from build123d import *

# Parameters (mm, degrees)
SKETCH2_R             = 6.35
SKETCH2_R_2           = 3.81
BOSS_EXTRUDE1_DEPTH   = 34.925
BOSS_EXTRUDE1_2_DEPTH = 34.925
BOSS_EXTRUDE1_3_DEPTH = 34.925
BOSS_EXTRUDE1_4_DEPTH = 34.925
SKETCH1_R             = 77.4954
SKETCH1_R_2           = 57.15
BOSS_EXTRUDE2_DEPTH   = 3.175
SKETCH3_R             = 3.81
CUT_EXTRUDE1_DEPTH    = 4.175
FILLET1_R             = 2.54


with BuildPart() as part:
    # Sketch2 → Boss-Extrude1 (new body)
    with BuildSketch(Plane(origin=(0, -40.33266, 0), x_dir=(1, 0, 0), z_dir=(0, 1, 0))):
        with Locations((-38.1, 56.870055469)):
            Circle(SKETCH2_R)
        with Locations((-38.1, 56.870055469)):
            Circle(SKETCH2_R_2, mode=Mode.SUBTRACT)
    extrude(amount=BOSS_EXTRUDE1_DEPTH)



with BuildPart() as body_2:
    # Sketch2 → Boss-Extrude1 2 (new body)
    with BuildSketch(Plane(origin=(0, -40.33266, 0), x_dir=(1, 0, 0), z_dir=(0, 1, 0))):
        with Locations((38.1, 56.870055469)):
            Circle(SKETCH2_R)
        with Locations((38.1, 56.870055469)):
            Circle(SKETCH2_R_2, mode=Mode.SUBTRACT)
    extrude(amount=BOSS_EXTRUDE1_2_DEPTH)


with BuildPart() as body_3:
    # Sketch2 → Boss-Extrude1 3 (new body)
    with BuildSketch(Plane(origin=(0, -40.33266, 0), x_dir=(1, 0, 0), z_dir=(0, 1, 0))):
        with Locations((38.1, -56.870055469)):
            Circle(SKETCH2_R)
        with Locations((38.1, -56.870055469)):
            Circle(SKETCH2_R_2, mode=Mode.SUBTRACT)
    extrude(amount=BOSS_EXTRUDE1_3_DEPTH)


with BuildPart() as body_4:
    # Sketch2 → Boss-Extrude1 4 (new body)
    with BuildSketch(Plane(origin=(0, -40.33266, 0), x_dir=(1, 0, 0), z_dir=(0, 1, 0))):
        with Locations((-38.1, -56.870055469)):
            Circle(SKETCH2_R)
        with Locations((-38.1, -56.870055469)):
            Circle(SKETCH2_R_2, mode=Mode.SUBTRACT)
    extrude(amount=BOSS_EXTRUDE1_4_DEPTH)


with BuildPart() as part_1:
    add(part.part)

    add(body_2.part)  # Boss-Extrude2 merges body 2

    add(body_3.part)  # Boss-Extrude2 merges body 3

    add(body_4.part)  # Boss-Extrude2 merges body 4
    # Sketch1 → Boss-Extrude2 (add)
    with BuildSketch(Plane(origin=(0, -40.33266, 0), x_dir=(1, 0, 0), z_dir=(0, 1, 0))):
        Circle(SKETCH1_R)
        Circle(SKETCH1_R_2, mode=Mode.SUBTRACT)
    extrude(amount=-BOSS_EXTRUDE2_DEPTH)

    # Sketch3 → Cut-Extrude1 (cut, through all)
    with BuildSketch(Plane(origin=(0, -40.33266, 0), x_dir=(1, 0, 0), z_dir=(0, 1, 0))):
        with Locations((-38.1, -56.870055469)):
            Circle(SKETCH3_R)
        with Locations((38.1, -56.870055469)):
            Circle(SKETCH3_R)
        with Locations((38.1, 56.870055469)):
            Circle(SKETCH3_R)
        with Locations((-38.1, 56.870055469)):
            Circle(SKETCH3_R)
    extrude(amount=-CUT_EXTRUDE1_DEPTH, mode=Mode.SUBTRACT)

    # Fillet1
    fillet1_edges = [part_1.edges().sort_by_distance(p)[0] for p in [
        (-44.45, -40.33266, -56.870055469),
        (31.75, -40.33266, -56.870055469),
        (31.75, -40.33266, 56.870055469),
        (-44.45, -40.33266, 56.870055469),
    ]]
    fillet(fillet1_edges, radius=FILLET1_R)


solid = part_1.part
CAD build for the part. Positions are in the model's coordinates, mm. A direction names the side the tool comes from. Coordinates: 2 decimals unless noted, no trailing zeros. Write each loop counter-clockwise with the first axis right and the second up, starting at its lowest first coordinate (ties: lowest second). Pieces come first, ordered by that corner, then holes. Notation, with made-up numbers: (24.5, 0.25) - (78.5, 0.25) arc R21 ccw to (78.5, 21.25) - close; hole circle Ø6 at (-0.75, 81.25). An arc over 180 degrees is marked (long way). Use a Markdown table: item, result. Add a question column.
Item 1: Mould opens along X. For faces 1 (the face through (-57.117, -41.898, -52.375)), 2 (the face through (33.42, -21.83, -61.16)), 3 (the face through (41, -5.408, 60)) say: pulls with the +X half, pulls with the -X half, needs draft (parallel to the pull), parting line crosses it, or undercut.
Item 2: Band-saw the part on A-A, the plane z = 0. Give the cut face in (x, y).
Item 3: Band-saw the part on C-C, the plane y = -17.5. Give the cut face in (x, z), and give its area (3 significant figures).
Item 4: Band-saw the part on B-B, the plane x = 0. Give the cut face in (y, z), and give its area (3 significant figures).
Item 5: Drill centre lines: L1, parallel to Z at x = 38, y = -19; L2, parallel to Z at x = 38.1, y = -42.6; L3, parallel to X at y = -19, z = 58. Where is each one in solid material? Low to high. Write a range as from..to.
Item 6: 3-axis set-ups, long thin cutter, end or side, ignore diameter. For faces 4 (the face through (-57.095, -41.898, -2.513)), 5 (the face through (33.06, -21.83, 60.73)): which of +Z, -Z, +X, -X, +Y, -Y reach the whole face in a straight line?
Item 7: Band-saw the part on D-D, the plane x = 38.1. Give the cut face in (y, z), and give its area (3 significant figures).
Item 8: Flat gauge pins, fed straight in: pin 1 (10 mm diameter, centred on x = -40.5, y = -12, fed in from +Z); pin 2 (12 mm diameter, centred on x = 20, y = -24, fed in from +Z); pin 3 (8 mm diameter, centred on x = -24, y = -38.5, fed in from +Z); pin 4 (3 mm diameter, centred on y = -33.5, z = -49.5, fed in from -X). Where does each tip first touch, or does it go through?
Numbers:
| question | item | result |
|---|---|---|
| 1 | face 1 | parting line crosses it |
| 1 | face 2 | undercut |
| 1 | face 3 | needs draft |
| 2 | outline | (-77.5, -43.51) - (-57.15, -43.51) - (-57.15, -40.33) - (-77.5, -40.33) - close; (57.15, -43.51) - (77.5, -43.51) - (77.5, -40.33) - (57.15, -40.33) - close |
| 3 | outline | circle Ø12.7 at (-38.1, -56.87); circle Ø12.7 at (-38.1, 56.87); circle Ø12.7 at (38.1, -56.87); circle Ø12.7 at (38.1, 56.87); hole circle Ø7.62 at (-38.1, -56.87); hole circle Ø7.62 at (-38.1, 56.87); hole circle Ø7.62 at (38.1, -56.87); hole circle Ø7.62 at (38.1, 56.87) |
| 3 | area | 324 mm2 |
| 4 | outline | (-43.51, -77.5) - (-40.33, -77.5) - (-40.33, -57.15) - (-43.51, -57.15) - close; (-43.51, 57.15) - (-40.33, 57.15) - (-40.33, 77.5) - (-43.51, 77.5) - close |
| 4 | area | 129 mm2 |
| 5 | L1 | -63.22..-60.68, -53.06..-50.52, 50.52..53.06, 60.68..63.22 |
| 5 | L2 | -67.48..-60.68, -53.06..-42.6, 42.6..53.06, 60.68..67.48 |
| 5 | L3 | -44.35..-41.74, -34.46..-31.85, 31.85..34.46, 41.74..44.35 |
| 6 | face 4 | +Y, -Y |
| 6 | face 5 | +Y |
| 7 | outline | (-43.51, -67.48) - (-40.33, -67.48) - (-40.33, -65.76) arc R2.54 cw to (-37.79, -63.22) - (-5.41, -63.22) - (-5.41, -60.68) - (-43.51, -60.68) - close; (-43.51, -53.06) - (-5.41, -53.06) - (-5.41, -50.52) - (-37.79, -50.52) arc R2.54 cw to (-40.33, -47.98) - (-40.33, -42.6) - (-43.51, -42.6) - close; (-43.51, 42.6) - (-40.33, 42.6) - (-40.33, 47.98) arc R2.54 cw to (-37.79, 50.52) - (-5.41, 50.52) - (-5.41, 53.06) - (-43.51, 53.06) - close; (-43.51, 60.68) - (-5.41, 60.68) - (-5.41, 63.22) - (-37.79, 63.22) arc R2.54 cw to (-40.33, 65.76) - (-40.33, 67.48) - (-43.51, 67.48) - close |
| 7 | area | 470 mm2 |
| 8 | pin 1 | z = 63.22 |
| 8 | pin 2 | through |
| 8 | pin 3 | z = 74.75 |
| 8 | pin 4 | x = -40.52 |
